The drawing under review shows one solid part. Ordinate dimensions are in mm from its lowest x, y, z. A direction names the side the tool comes from. Coordinates: 2 decimals unless noted, no trailing zeros. Order: outer loops, then holes, each group sorted by start corner. A loop starts at its lowest first (then second) coordinate and runs counter-clockwise, first axis right, second up.
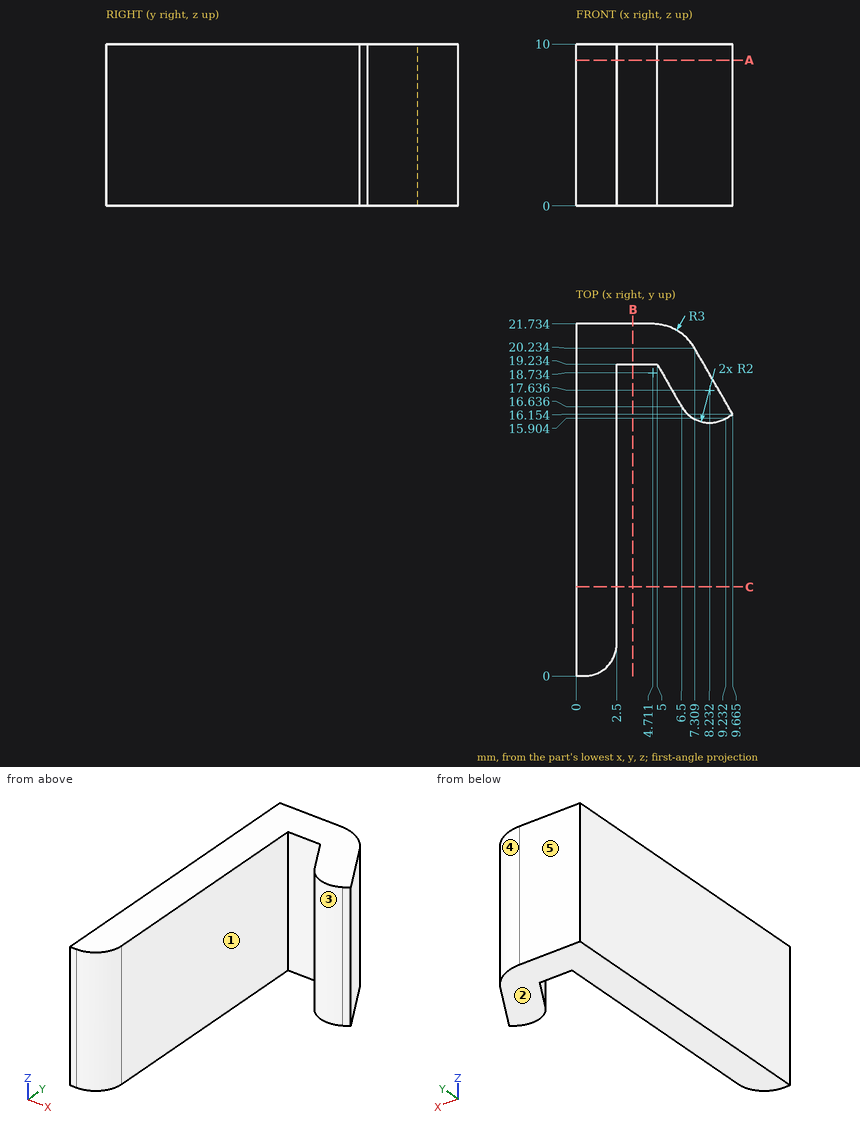
(1) We need section C-C, the plane y = 5.5. Write out the cut boundary in (x, z).
A:
outline: (0, 0) - (2.5, 0) - (2.5, 10) - (0, 10) - close
(2) We need section B-B, the plane x = 3.5. Write out the cut boundary in (y, z), and give its area (3 significant figures).
A:
outline: (19.23, 0) - (21.73, 0) - (21.73, 10) - (19.23, 10) - close
area: 25.0 mm2
(3) We need section A-A, the plane z = 9. Write out the cut boundary in (x, y) (1 decimal).
A:
outline: (0, 0) - (0.5, 0) arc R2 ccw to (2.5, 2) - (2.5, 19.2) - (5, 19.2) - (6.5, 16.6) arc R2 ccw to (9.2, 15.9) - (9.7, 16.2) - (7.3, 20.2) arc R3 ccw to (4.7, 21.7) - (0, 21.7) - close
(4) Draft analysis for pull direction X (two halves, no side actions). For the marked faces 3, 4 and 5, state which applies: released by +X, released by -X, zero draft, split by the parting line, or undercut.
A:
face 3: undercut
face 4: released by +X
face 5: zero draft
(5) Wall thickness on probe 1 along X at (y, z) = (13.5, 0.5); probe 2 along Y at (x, z) = (4.25, 2.5); probe 3 along X at (y, z) = (17, 0.75) (1 decimal): over which ranges is each line inside the solid? List them lowest first.
A:
probe 1: x = 0 to 2.5
probe 2: y = 19.23 to 21.73
probe 3: x = 0 to 2.5, 6.3 to 9.2
(6) Machinability: for the marked faces 1 and 2, which of the approach directions +Z, -Z, +X, -X, +Y, -Y give a long, thin tool a straight path to every point of the face, cutting with its end or side? Answer none if there is none.
A:
face 1: +Z, -Z, -Y
face 2: -Z, +X, -X, +Y, -Y
(7) For pin 1 Ø6 at (y, z) = (7, 4.5) entering from +X; pin 2 Ø1.5 at (x, z) = (2, 7.5) entering from -Y; pin 3 Ø4 at (x, y) = (6, 12.5) entering from +Z, all flat-tipped, find the tip position at first contact; note any pin that passes through.
A:
pin 1: stops at x = 2.5
pin 2: stops at y = 0.15
pin 3: passes through
